Geometry: final body of the model. Coordinates: model frame, mm. Give positions to 0.01 mm unless a question says otherwise; leave off trailing zeros. Write each loop counter-clockwise with the first axis right and the second up, starting at its lowest first coordinate (ties: lowest second). Pieces come first, ordered by that corner, then holes. Notation, with made-up numbers: (18.5, 25) -> (24.5, 25) arc R27 ccw to (24.5, 49) -> close; hole circle Ø3 at (-24.75, 38.5). An arc over 180 degrees is marked (long way). Use CSV: the item, a comma, the result in double quotes. Start each with the question number.
1) Section C-C (x = -27). Output: boundary loops of the cut face in (y, z).
2) Draft query along Y for faces 1 (the face through (-34.32, 0, -20.25)), 2 (the face through (-34.32, 19.05, -20.25)), 3 (the face through (-42.845, 12.624, -0.688)). Return one class per face: pulls with the +Y half, pulls with the -Y half, needs draft (parallel to the pull), parting line crosses it, or undercut.
3) Material intervals for line 1 (Y direction, x = 43.75, z = 0); line 2 (Z direction, x = 29.5, y = 7.5); line 3 (X direction, y = 10.5, z = 25), sorted ascending. Write a range as [from, to].
4) Section A-A (x = 0). Output: boundary loops of the cut face in (y, z).
5) Section B-B (z = 0). Output: boundary loops of the cut face in (x, y).
6) Section D-D (z = -33). Output: boundary loops of the cut face in (x, y), plus the area to 3 significant figures.
7) Contact query for flat-ended pins moving along their axis: P1, Ø1.5, axis at x = 14.5, y = 13.5, coming from the -Z side; P2, Ø12, axis at x = -2.5, z = 28, coming from the +Y side; P3, Ø3, axis at y = 4.5, z = -29, coming from the -X side; P4, Ø3, axis at x = -34, y = 9.5, coming from the +Z side. Output: stop coordinate, or through.
```python
from build123d import *

# Parameters (mm, degrees)
SKETCH1_R               = 46.0375
SKETCH1_R_2             = 39.6875
BOSS_EXTRUDE1_DEPTH     = 19.05
CUT_EXTRUDE4_DEPTH      = 76.2
CUT_EXTRUDE4_DEPTH_BACK = 76.2
SKETCH7_R               = 3.175
CUT_EXTRUDE5_DEPTH      = 76.2
CUT_EXTRUDE5_DEPTH_BACK = 76.2
SKETCH10_R              = 3.175


with BuildPart() as part:
    # Sketch1 → Boss-Extrude1 (new body)
    with BuildSketch(Plane(origin=(0, 0, 0), x_dir=(1, 0, 0), z_dir=(0, 1, 0))):
        with Locations(Location((0, 0, 0), (0, 0, 90))):
            Circle(SKETCH1_R)
        with Locations(Location((0, 0, 0), (0, 0, 90))):
            Circle(SKETCH1_R_2, mode=Mode.SUBTRACT)
    extrude(amount=BOSS_EXTRUDE1_DEPTH)

    # Sketch7 → Cut-Extrude4 (cut, two sides: drawn at the far end of the back side and taken through both)
    with BuildSketch(Plane.XY.offset(-CUT_EXTRUDE4_DEPTH_BACK)):
        with Locations(Location((0, 9.525, 0), (0, 0, 180))):
            Circle(SKETCH7_R)
    extrude(amount=CUT_EXTRUDE4_DEPTH + CUT_EXTRUDE4_DEPTH_BACK, mode=Mode.SUBTRACT)

    # Sketch10 → Cut-Extrude5 (cut, two sides: drawn at the far end of the back side and taken through both)
    with BuildSketch(Plane(origin=(0, 0, 0), x_dir=(0, 0, -1), z_dir=(1, 0, 0)).offset(-CUT_EXTRUDE5_DEPTH_BACK)):
        with Locations(Location((0, 9.525, 0), (0, 0, 180))):
            Circle(SKETCH10_R)
    extrude(amount=CUT_EXTRUDE5_DEPTH + CUT_EXTRUDE5_DEPTH_BACK, mode=Mode.SUBTRACT)


solid = part.part
```
Answers follow:
1,outline,"(0, -37.29) -> (19.05, -37.29) -> (19.05, -29.09) -> (0, -29.09) -> close; (0, 29.09) -> (19.05, 29.09) -> (19.05, 37.29) -> (0, 37.29) -> close"
2,face 1,"pulls with the -Y half"
2,face 2,"pulls with the +Y half"
2,face 3,"undercut"
3,line 1,"y = [0, 6.35], [12.7, 19.05]"
3,line 2,"z = [-35.34, -26.55], [26.55, 35.34]"
3,line 3,"x = [-38.66, -30.82], [30.82, 38.66]"
4,outline,"(0, -46.04) -> (6.35, -46.04) -> (6.35, -39.69) -> (0, -39.69) -> close; (0, 39.69) -> (6.35, 39.69) -> (6.35, 46.04) -> (0, 46.04) -> close; (12.7, -46.04) -> (19.05, -46.04) -> (19.05, -39.69) -> (12.7, -39.69) -> close; (12.7, 39.69) -> (19.05, 39.69) -> (19.05, 46.04) -> (12.7, 46.04) -> close"
5,outline,"(-46.04, 0) -> (-39.69, 0) -> (-39.69, 6.35) -> (-46.04, 6.35) -> close; (-46.04, 12.7) -> (-39.69, 12.7) -> (-39.69, 19.05) -> (-46.04, 19.05) -> close; (39.69, 0) -> (46.04, 0) -> (46.04, 6.35) -> (39.69, 6.35) -> close; (39.69, 12.7) -> (46.04, 12.7) -> (46.04, 19.05) -> (39.69, 19.05) -> close"
6,outline,"(-32.1, 0) -> (-22.05, 0) -> (-22.05, 19.05) -> (-32.1, 19.05) -> close; (22.05, 0) -> (32.1, 0) -> (32.1, 19.05) -> (22.05, 19.05) -> close"
6,area,"383 mm^2"
7,P1,"stops at z = -43.94"
7,P2,"passes through"
7,P3,"stops at x = -36.92"
7,P4,"stops at z = 32.61"
